Source: three-view drawing plus pictorial views. Frame: mm from the lowest corner of the part. Give positions to 0.01 mm unless a question says otherwise; leave off trailing zeros. Write each loop counter-clockwise with the first axis right and the second up, starting at its lowest first coordinate (ties: lowest second). Pieces come first, ordered by that corner, then holes.
Q1. Line query: L1, parallel to X at y = 0.4, z = 2.75; L2, parallel to Z at x = 27.25, y = 0.3. Output: solid intervals per line, ascending.
Q2. Cut plane C-C on x = 26.9. Return the cut outline in (y, z), plus the area to 3 significant figures.
Q3. Cut plane A-A on y = 0.7. Return the cut outline in (x, z).
Q4. Pin query (flat end, axial travel): pin 1 (2.5 mm diameter, centred on x = 26.9, z = 2.75, fed in from -Y). Return the tip coordinate at first contact, or that it passes through.
Q5. Cut plane B-B on z = 2.75. Return the cut outline in (x, y), plus the area to 3 significant figures.
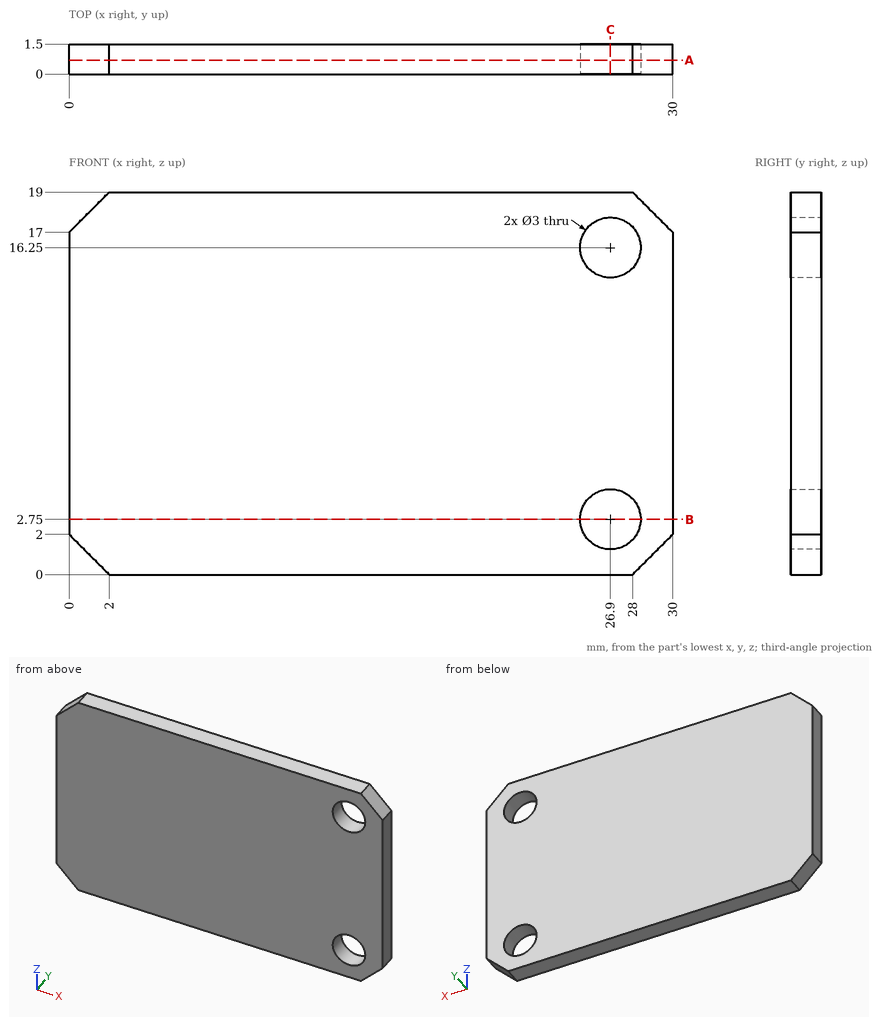
Data:
1. L1: x = 0 to 25.4, 28.4 to 30
1. L2: z = 0 to 1.29, 4.21 to 14.79, 17.71 to 19
2. outline: (0, 0) - (1.5, 0) - (1.5, 1.25) - (0, 1.25) - close; (0, 4.25) - (1.5, 4.25) - (1.5, 14.75) - (0, 14.75) - close; (0, 17.75) - (1.5, 17.75) - (1.5, 19) - (0, 19) - close
2. area: 19.5 mm2
3. outline: (0, 2) - (2, 0) - (28, 0) - (30, 2) - (30, 17) - (28, 19) - (2, 19) - (0, 17) - close; hole circle Ø3 at (26.9, 2.75); hole circle Ø3 at (26.9, 16.25)
4. pin 1: passes through
5. outline: (0, 0) - (25.4, 0) - (25.4, 1.5) - (0, 1.5) - close; (28.4, 0) - (30, 0) - (30, 1.5) - (28.4, 1.5) - close
5. area: 40.5 mm2
